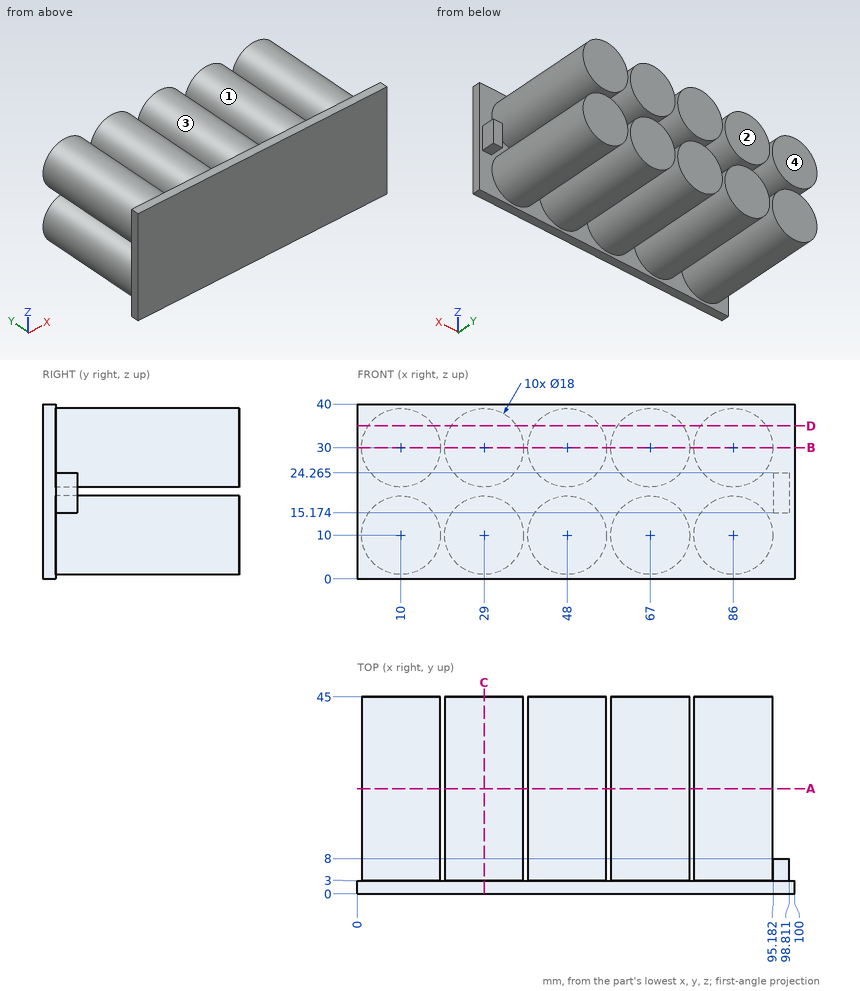
Input: dimensioned drawing with shaded views. Units: mm. Origin: part minimum x, y, z. A direction names the side the tool comes from. Give positions to 0.01 mm unless a question says otherwise; leave off trailing zeros. Write each loop counter-clockwise with the first axis right and the second up, starting at its lowest first coordinate (ties: lowest second). Pieces come first, ordered by that corner, then holes. Notation, with made-up numbers: (15.5, 32) - (24.5, 32) arc R15 cw to (24.5, 40) - close; hole circle Ø2 at (47, -35). An arc over 180 degrees is marked (long way). Write item = value, one per line. Start each with the question number.
1) Pin query (flat end, axial travel): pin 1 (4 mm diameter, centred on x = 85.5, y = 25, fed in from -Z); pin 2 (1.8 mm diameter, centred on x = 96.5, y = 4.5, fed in from +Z) (1 decimal); pin 3 (5 mm diameter, centred on y = 36, z = 25.5, fed in from -X) (1 decimal); pin 4 (20 mm diameter, centred on x = 57.5, z = 18.5, fed in from +Y). Return the tip coordinate at first contact, or that it passes through.
2) Cut plane A-A (y = 24). Give the number of separate pieces and of enclosed holes in the cut face.
3) Draft query along Z for the marked faces 1 and 2. Return one class per face: pulls with the +Z half, pulls with the -Z half, needs draft (parallel to the pull), parting line crosses it, or undercut.
4) Material intervals for L1, parallel to X at y = 36, z = 30.5; L2, parallel to X at y = 3.5, z = 37 (1 decimal); L3, parallel to Z at x = 28.5, y = 14, sorted ascending. Write a range as [from, to].
5) Cut plane D-D (z = 35). Return loops of the section in (x, y), and give its area (3 significant figures).
6) Cut plane C-C (x = 29). Return loops of the section in (y, z), and give its area (3 significant figures).
7) Cut plane B-B (z = 30). Return loops of the section in (x, y).
8) Reachability of the marked faces 3 and 4 from +Z, -Z, +X, -X, +Y, -Y: full face, straight path, thin tool, end or side. Return the list, or none.
Answers follow:
q1.pin_1 = 1
q1.pin_2 = 24.3
q1.pin_3 = 1.2
q1.pin_4 = 45
q2.separate_pieces = 10
q2.enclosed_holes = 0
q3.face_1 = undercut
q3.face_2 = needs draft
q4.L1 = [1.01, 18.99], [20.01, 37.99], [39.01, 56.99], [58.01, 75.99], [77.01, 94.99]
q4.L2 = [4.3, 15.7], [23.3, 34.7], [42.3, 53.7], [61.3, 72.7], [80.3, 91.7]
q4.L3 = [1.01, 18.99], [21.01, 38.99]
q5.outline = (0, 0) - (100, 0) - (100, 3) - (93.48, 3) - (93.48, 45) - (78.52, 45) - (78.52, 3) - (74.48, 3) - (74.48, 45) - (59.52, 45) - (59.52, 3) - (55.48, 3) - (55.48, 45) - (40.52, 45) - (40.52, 3) - (36.48, 3) - (36.48, 45) - (21.52, 45) - (21.52, 3) - (17.48, 3) - (17.48, 45) - (2.52, 45) - (2.52, 3) - (0, 3) - close
q5.area = 3,440 mm^2
q6.outline = (0, 0) - (3, 0) - (3, 1) - (45, 1) - (45, 19) - (3, 19) - (3, 21) - (45, 21) - (45, 39) - (3, 39) - (3, 40) - (0, 40) - close
q6.area = 1,630 mm^2
q7.outline = (0, 0) - (100, 0) - (100, 3) - (95, 3) - (95, 45) - (77, 45) - (77, 3) - (76, 3) - (76, 45) - (58, 45) - (58, 3) - (57, 3) - (57, 45) - (39, 45) - (39, 3) - (38, 3) - (38, 45) - (20, 45) - (20, 3) - (19, 3) - (19, 45) - (1, 45) - (1, 3) - (0, 3) - close
q8.face_3 = +Y
q8.face_4 = +Z, -Z, +X, -X, +Y
